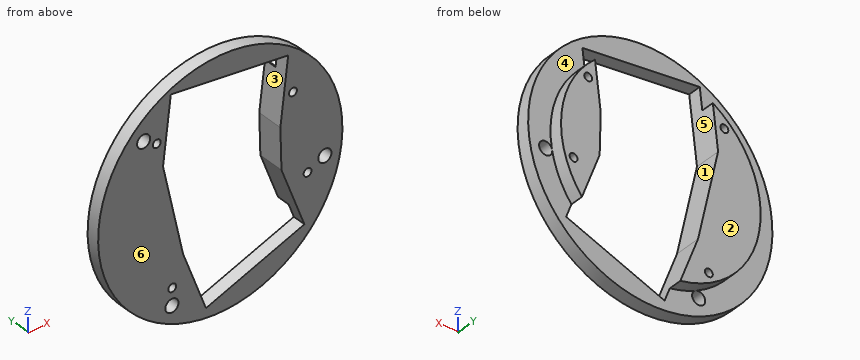
from build123d import *

# Parameters (mm, degrees)
ESQUISSE1_R             = 46.5
BOSS_EXTRU_1_DEPTH      = 5
ESQUISSE3_R             = 38
BOSS_EXTRU_2_DEPTH      = 5
ESQUISSE4_R             = 2.5
ENL_V_MAT_EXTRU_1_DEPTH = 6
ESQUISSE5_R             = 1.5
ENL_V_MAT_EXTRU_2_DEPTH = 11
ENL_V_MAT_EXTRU_4_DEPTH = 11
ENL_V_MAT_EXTRU_5_DEPTH = 11
ENL_V_MAT_EXTRU_6_DEPTH = 11


with BuildPart() as part:
    # Esquisse1 → Boss.-Extru.1 (new body)
    with BuildSketch(Plane(origin=(0, 0, 0), x_dir=(1, 0, 0), z_dir=(0, 1, 0))):
        with Locations(Location((-2.835211314, 0, 0), (0, 0, 270))):  # turned: the seam where the file's is
            Circle(ESQUISSE1_R)
    extrude(amount=BOSS_EXTRU_1_DEPTH)

    # Esquisse3 → Boss.-Extru.2 (add)
    with BuildSketch(Plane(origin=(0, 5, 0), x_dir=(1, 0, 0), z_dir=(0, 1, 0))):
        with Locations(Location((-2.835211314, 0, 0), (0, 0, 270))):  # turned: the seam where the file's is
            Circle(ESQUISSE3_R)
    extrude(amount=BOSS_EXTRU_2_DEPTH)

    # Esquisse4 → Enlèv. mat.-Extru.1 (cut, through all)
    with BuildSketch(Plane(origin=(0, 5, 0), x_dir=(1, 0, 0), z_dir=(0, 1, 0))):
        with Locations(Location((-21.248861584, 36.049258979, 0), (0, 0, 270))):  # turned: the seam where the file's is
            Circle(ESQUISSE4_R)
        with Locations(Location((36.99885245, 7.201316076, 0), (0, 0, 270))):  # turned: the seam where the file's is
            Circle(ESQUISSE4_R)
        with Locations(Location((-32.01877618, -28.052292793, 0), (0, 0, 270))):  # turned: the seam where the file's is
            Circle(ESQUISSE4_R)
    extrude(amount=-ENL_V_MAT_EXTRU_1_DEPTH, mode=Mode.SUBTRACT)

    # Esquisse5 → Enlèv. mat.-Extru.2 (cut, through all)
    with BuildSketch(Plane(origin=(0, 10, 0), x_dir=(1, 0, 0), z_dir=(0, 1, 0))):
        with Locations(Location((-27.01877618, -25.04959308, 0), (0, 0, 270))):  # turned: the seam where the file's is
            Circle(ESQUISSE5_R)
        with Locations(Location((24.833784646, -21.136546209, 0), (0, 0, 270))):  # turned: the seam where the file's is
            Circle(ESQUISSE5_R)
        with Locations(Location((30.401495955, 10.375365678, 0), (0, 0, 270))):  # turned: the seam where the file's is
            Circle(ESQUISSE5_R)
        with Locations(Location((-21.116944618, 29.632839055, 0), (0, 0, 270))):  # turned: the seam where the file's is
            Circle(ESQUISSE5_R)
    extrude(amount=-ENL_V_MAT_EXTRU_2_DEPTH, mode=Mode.SUBTRACT)

    # Esquisse6 → Enlèv. mat.-Extru.4 (cut, through all)
    with BuildSketch(Plane(origin=(0, 10, 0), x_dir=(1, 0, 0), z_dir=(0, 1, 0))):
        Polygon((-17.016589785, 19.158599311), (-8.28612786, 42.584632577), (29.195500656, 28.615902705), (20.465038731, 5.189869439), align=None)
    extrude(amount=-ENL_V_MAT_EXTRU_4_DEPTH, mode=Mode.SUBTRACT)

    # Esquisse7 → Enlèv. mat.-Extru.5 (cut, through all)
    with BuildSketch(Plane(origin=(0, 10, 0), x_dir=(1, 0, 0), z_dir=(0, 1, 0))):
        Polygon((-24.638086397, -15.703679396), (-21.665671556, -40.526345449), (23.01512734, -35.175998737), (20.0427125, -10.353332683), align=None)
    extrude(amount=-ENL_V_MAT_EXTRU_5_DEPTH, mode=Mode.SUBTRACT)

    # Esquisse8 → Enlèv. mat.-Extru.6 (cut, through all)
    with BuildSketch(Plane(origin=(0, 10, 0), x_dir=(1, 0, 0), z_dir=(0, 1, 0))):
        Polygon((-17.016589785, 19.158599311), (-24.638086397, -15.703679396), (20.0427125, -10.353332683), (20.465038731, 5.189869439), align=None)
    extrude(amount=-ENL_V_MAT_EXTRU_6_DEPTH, mode=Mode.SUBTRACT)


solid = part.part
Geometry check sheet. Reference: the model listing, model coordinates, mm. Face numbers are marked on the shaded views. A direction names the side the tool comes from. Give positions to 0.01 mm unless a question says otherwise; leave off trailing zeros. Write each loop counter-clockwise with the first axis right and the second up, starting at its lowest first coordinate (ties: lowest second). Pieces come first, ordered by that corner, then holes.
1) Cross-section at D-D (y = 2.75). Count the separate pieces of the cut face and the enclosed holes in it, plus the area to 3 significant figures.
Values follow:
separate pieces: 1
enclosed holes: 8
area: 3,530 mm2
2) Thickness scan on line 1 (X direction, y = 4, z = 21.5); line 2 (X direction, y = 6.75, z = 21.5); line 3 (X direction, y = 7.5, z = 19). Record the ranges inside material, lowest first.
Values follow:
line 1: x = -44.07 to -23.94, 21.38 to 23.38, 26.29 to 38.4
line 2: x = -34.17 to -23.94, 21.38 to 23.38, 26.29 to 28.5
line 3: x = -35.74 to -24.24, 21.08 to 30.07
3) Set-up check for the marked faces 4, 5 and 6: record each of +Z, -Z, +X, -X, +Y, -Y from which the full face is reachable in a straight line by a thin tool's end or side.
Values follow:
face 4: +Y
face 5: +Y, -Y
face 6: +Z, -Z, +X, -X, -Y
4) Go/stop test with flat-tipped pins: pin 1 Ø1 at (y, z) = (4.5, 23.5) entering from +X; pin 2 Ø1.8 at (x, z) = (-27.02, 25.05) entering from -Y; pin 3 Ø5 at (y, z) = (5, -26) entering from -X; pin 4 Ø5 at (x, y) = (22.5, 3.5) entering from +Z. Record where each tip stops, or that it passes through.
Values follow:
pin 1: stops at x = 37.58
pin 2: passes through
pin 3: stops at x = -42.96
pin 4: stops at z = 40.51
5) Cross-section at C-C (x = 10.5). Record the boundary of the cut face in (y, z).
Values follow:
outline: (0, -44.55) - (5, -44.55) - (5, -35.58) - (0, -35.58) - close; (0, 36.67) - (5, 36.67) - (5, 44.55) - (0, 44.55) - close
6) Cross-section at A-A (y = 7.75). Record the boundary of the cut face in (x, z), plus the area to 3 significant figures.
Values follow:
outline: (-24.64, 15.7) - (-22.63, 32.43) arc R38 ccw to (-10.27, -37.27) - (-17.02, -19.16) - close; (20.04, 10.35) - (20.47, -5.19) - (27.2, -23.27) arc R38 ccw to (22.22, 28.57) - close; hole circle Ø3 at (-27.02, 25.05); hole circle Ø3 at (-21.12, -29.63); hole circle Ø3 at (24.83, 21.14); hole circle Ø3 at (30.4, -10.38)
area: 1,510 mm2
7) Release check for a two-part mould opening along X. For the marked faces 1, 2 and 3 record: released by +X, released by -X, zero draft, split by the parting line, or undercut.
Values follow:
face 1: undercut
face 2: zero draft
face 3: undercut
8) Cross-section at B-B (z = 0). Record the boundary of the cut face in (x, y) (3 decimals).
Values follow:
outline: (-49.335, 0) - (-21.205, 0) - (-21.205, 10) - (-40.835, 10) - (-40.835, 5) - (-49.335, 5) - close; (20.324, 0) - (43.665, 0) - (43.665, 5) - (35.165, 5) - (35.165, 10) - (20.324, 10) - close
